CAD build for the part. Positions are in the model's coordinates, mm. Face numbers are marked on the shaded views. A direction names the side the tool comes from. Round coordinates to 2 decimals unless told otherwise and drop trailing zeros. Order: outer loops, then holes, each group sorted by start corner. A loop starts at its lowest first (then second) coordinate and runs counter-clockwise, first axis right, second up. Notation, with made-up numbers: M 12,-22 L 26,-22 A21 ccw 26,9 Z; hole C -25,-25 d11. An arc over 180 degrees is marked long. Put each result on its own line as item: value.
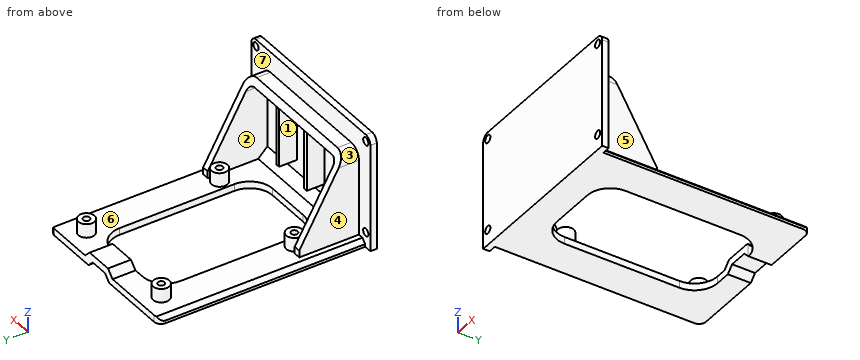
Autodesk Fusion 360 part; units mm, degrees
sketch "Sketch3" plane through (0, 0, 0) normal (0, 1, 0) x (1, 0, 0)
  line L0 (-39, -50) -> (39, -50)
  line L1 (39, -50) -> (39, 0)
  line L2 (39, 0) -> (-39, 0)
  line L3 (-39, 0) -> (-39, -50)
  line L4 (-56.129, 0) -> (56.129, 0) construction
  circle A0 centre (-36, -47) radius 1.7
  circle A1 centre (-36, -47) radius 3
  circle A2 centre (36, -47) radius 1.7
  circle A3 centre (36, -47) radius 3
  circle A4 centre (-36, -6.7) radius 1.7
  circle A5 centre (-36, -6.7) radius 3
  circle A6 centre (36, -6.7) radius 1.7
  circle A7 centre (36, -6.7) radius 3
  line L5 (-39, -5) -> (39, -5) construction
  dimension "d32" = 50
  dimension "d33" = 78
  dimension "d34" = 39
  dimension "d35" = 3.4
  dimension "d36" = 6
  dimension "d37" = 3.4
  dimension "d38" = 6
  dimension "d39" = 3.4
  dimension "d40" = 6
  dimension "d41" = 3.4
  dimension "d42" = 6
  dimension "d43" = 5
extrude "Extrude3" add sketch "Sketch3" along normal blind 3 contours A7 | A5 | L0 L1 L2 L3 A1 A3 | A1 | A3
sketch "Sketch4" plane through (0, 3, 0) normal (0, 1, 0) x (-1, 0, 0)
  circle A0 centre (36, 47) radius 1.7
  circle A1 centre (36, 6.7) radius 1.7
  circle A2 centre (-36, 47) radius 1.7
  circle A3 centre (-36, 6.7) radius 1.7
  line L0 (36, 50) -> (-36, 50)
  arc A4 (-36, 50) -> (-39, 47) centre (-36, 47) ccw
  line L1 (-39, 47) -> (-39, 0)
  line L2 (-39, 0) -> (39, 0)
  line L3 (39, 0) -> (39, 47)
  arc A5 (39, 47) -> (36, 50) centre (36, 47) ccw
  line L4 (-39, 3) -> (39, 3) construction
  line L5 (-35.6, 3) -> (35.6, 3)
  line L6 (35.6, 3) -> (35.6, 0)
  line L7 (35.6, 0) -> (-35.6, 0)
  line L8 (-35.6, 0) -> (-35.6, 3)
  line L9 (0, 50) -> (0, 0) construction
  line L10 (35.6, 1.2) -> (33.8, 3)
  line L11 (35.6, 1.2) -> (38.7868, 1.2) construction
  line L12 (-35.6, 1.2) -> (-33.8, 3)
  line L13 (-35.6, 1.2) -> (-32.9375, 1.2) construction
  point P0 (0, 3)
  dimension "d46" = 3
  dimension "d47" = 71.2
  dimension "d48" = 135
  dimension "d49" = 1.2
  dimension "d50" = 45
  dimension "d51" = 1.2
extrude "Extrude4" add sketch "Sketch4" along normal blind 90 contours L2 L5 L6 L7 L8 L10 L12
sketch "Sketch5" plane through (0, 0, 3) normal (0, 0, 1) x (-1, 0, 0)
  line L0 (33.8, -3) -> (-33.8, -3)
  line L1 (-33.8, -3) -> (-33.8, -93)
  line L2 (-33.8, -93) -> (33.8, -93)
  line L3 (33.8, -93) -> (33.8, -3)
  line L4 (0, -3) -> (0, -93) construction
  circle A0 centre (24.5, -26.5) radius 1.45
  circle A1 centre (24.5, -26.5) radius 3.5
  circle A2 centre (24.5, -84.5) radius 1.45
  circle A3 centre (24.5, -84.5) radius 3.5
  circle A4 centre (-24.5, -26.5) radius 1.45
  circle A5 centre (-24.5, -26.5) radius 3.5
  circle A6 centre (-24.5, -84.5) radius 1.45
  circle A7 centre (-24.5, -84.5) radius 3.5
  line L5 (28, -3) -> (-28, -3)
  line L6 (-28, -3) -> (-28, -88) construction
  line L7 (-28, -88) -> (28, -88) construction
  line L8 (28, -88) -> (28, -3) construction
  line L9 (20, -13) -> (-20, -13)
  line L10 (-20, -13) -> (-20, -83)
  line L11 (-20, -83) -> (20, -83)
  line L12 (20, -83) -> (20, -13)
  line L13 (33.8, -48) -> (-33.8, -48) construction
  line L14 (-28.5, -3) -> (-31.5, -3)
  line L15 (-31.5, -3) -> (-31.5, -29)
  line L16 (-31.5, -29) -> (-28.5, -29)
  line L17 (-28.5, -29) -> (-28.5, -3)
  point P0 (0, -88)
  point P1 (-28, -3)
  point P2 (0, -13)
  point P3 (20, -48)
  point P4 (-33.8, -48)
  point P5 (33.8, -48)
  dimension "d54" = 2.9
  dimension "d55" = 7
  dimension "d56" = 2.9
  dimension "d57" = 7
  dimension "d58" = 2.9
  dimension "d59" = 7
  dimension "d60" = 2.9
  dimension "d61" = 7
  dimension "d62" = 58
  dimension "d63" = 49
  dimension "d64" = 23.5
  dimension "d70" = 56
  dimension "d71" = 85
  dimension "d86" = 70
  dimension "d87" = 70
  dimension "d88" = 40
  dimension "d159" = 3
  dimension "d160" = 26
  dimension "d161" = 7
extrude "Extrude8" add sketch "Sketch5" along normal blind 38 contours L0 L14 L15 L16 L17
chamfer "Chamfer4" distance 20 distance2 35 1 edges at (30, 29, 41) measured on face at (30.5, 11.6667, 41)
mirror "Mirror1" about plane through (0, 0, 0) normal (1, 0, 0) of "Extrude8"
extrude "Extrude7" cut sketch "Sketch5" against normal blind 3 contours L9 L10 L11 L12
extrude "Extrude5" add sketch "Sketch5" along normal blind 6 contours A1 | A3 | A5 | A7
fillet "Fillet1" radius 3 2 edges at (35.6, 93, 0.6) (-35.6, 93, 0.6)
sketch "Sketch7" plane through (0, 0, 0) normal (0, -1, 0) x (1, 0, 0)
  circle A0 centre (-36, 47) radius 1.7
  circle A1 centre (-36, 6.7) radius 1.7
  circle A2 centre (36, 47) radius 1.7
  circle A3 centre (36, 6.7) radius 1.7
  line L0 (36, 50) -> (-36, 50)
  arc A4 (-36, 50) -> (-39, 47) centre (-36, 47) ccw
  line L1 (-39, 47) -> (-39, 0)
  line L2 (-39, 0) -> (39, 0)
  line L3 (39, 0) -> (39, 47)
  arc A5 (39, 47) -> (36, 50) centre (36, 47) ccw
  line L4 (-28, 50) -> (-28, 0) construction
  line L5 (28, 50) -> (28, 0) construction
  line L6 (19, 50) -> (19, 48.3878)
  line L7 (-39, 3) -> (39, 3) construction
  line L8 (-21, 9) -> (-28, 9)
  line L9 (28, 9) -> (21, 9)
  point P0 (-24.5, 9)
  point P1 (24.5, 9)
  dimension "d72" = 11
  dimension "d73" = 11
  dimension "d74" = 3
fillet "Fillet2" radius 10 4 edges at (-20, 13, 1.5) (20, 13, 1.5) (-20, 83, 1.5) (20, 83, 1.5)
sketch "Sketch8" plane through (0, 0, 0) normal (0, 0, -1) x (1, 0, 0)
  line L0 (-10, -13) -> (10, -13)
  arc A0 (20, -23) -> (10, -13) centre (10, -23) ccw
  line L1 (20, -23) -> (20, -73)
  arc A1 (10, -83) -> (20, -73) centre (10, -73) ccw
  line L2 (10, -83) -> (-10, -83)
  arc A2 (-20, -73) -> (-10, -83) centre (-10, -73) ccw
  line L3 (-20, -73) -> (-20, -23)
  arc A3 (-10, -13) -> (-20, -23) centre (-10, -23) ccw
  arc A4 (-35.6, -90) -> (-32.6, -93) centre (-32.6, -90) ccw
  line L4 (-32.6, -93) -> (32.6, -93)
  arc A5 (32.6, -93) -> (35.6, -90) centre (32.6, -90) ccw
  line L5 (35.6, -90) -> (35.6, -3)
  line L6 (35.6, -3) -> (39, -3)
  line L7 (39, -3) -> (39, 0)
  line L8 (39, 0) -> (-39, 0)
  line L9 (-39, 0) -> (-39, -3)
  line L10 (-39, -3) -> (-35.6, -3)
  line L11 (-35.6, -3) -> (-35.6, -90)
  line L12 (3.6, -93) -> (3.6, -80.0711) construction
  line L13 (7.6, -93) -> (-0.4, -93)
  line L14 (-0.4, -93) -> (-0.4, -73.9514)
  line L15 (-0.4, -73.9514) -> (7.6, -73.9514)
  line L16 (7.6, -73.9514) -> (7.6, -93)
  dimension "d166" = 8
  dimension "d167" = 32
extrude "Extrude9" cut sketch "Sketch8" against normal blind 2.8 contours L2 L4 L13 L14 L16
sketch "Sketch11" plane through (0, 0, 3) normal (0, 0, 1) x (-1, 0, 0)
  line L0 (28.5, -29) -> (28.5, -3)
  line L1 (28.5, -3) -> (-28.5, -3)
  line L2 (-28.5, -3) -> (-28.5, -29)
  line L3 (-28.5, -29) -> (-31.5, -29)
  line L4 (-31.5, -29) -> (-31.5, -3)
  line L5 (-31.5, -3) -> (-33.8, -3)
  line L6 (-33.8, -3) -> (-33.8, -92.7495)
  arc A0 (-33.8, -92.7495) -> (-32.6, -93) centre (-32.6, -90) ccw
  line L7 (-32.6, -93) -> (32.6, -93)
  arc A1 (32.6, -93) -> (33.8, -92.7495) centre (32.6, -90) ccw
  line L8 (33.8, -92.7495) -> (33.8, -3)
  line L9 (33.8, -3) -> (31.5, -3)
  line L10 (31.5, -3) -> (31.5, -29)
  line L11 (31.5, -29) -> (28.5, -29)
  circle A2 centre (-24.5, -26.5) radius 3.5
  circle A3 centre (24.5, -26.5) radius 3.5
  line L12 (-10, -13) -> (10, -13)
  arc A4 (20, -23) -> (10, -13) centre (10, -23) ccw
  line L13 (20, -23) -> (20, -73)
  arc A5 (10, -83) -> (20, -73) centre (10, -73) ccw
  line L14 (10, -83) -> (-10, -83)
  arc A6 (-20, -73) -> (-10, -83) centre (-10, -73) ccw
  line L15 (-20, -73) -> (-20, -23)
  arc A7 (-10, -13) -> (-20, -23) centre (-10, -23) ccw
  circle A8 centre (24.5, -84.5) radius 3.5
  circle A9 centre (-24.5, -84.5) radius 3.5
  line L16 (-7.6, -83) -> (-7.6, -93)
  line L17 (0.4, -93) -> (0.4, -83)
  line L18 (-9.6, -83) -> (-9.6, -93)
  line L19 (2.4, -93) -> (2.4, -83)
  dimension "d170" = 2
  dimension "d171" = 2
extrude "Extrude10" add sketch "Sketch11" along normal blind 3 contours L7 L14 L17 L19 | L7 L14 L16 L17 | L7 L14 L16 L18
chamfer "Chamfer5" distance 3 angle 45 2 edges at (-2.4, 88, 3) (9.6, 88, 3)
chamfer "Chamfer6" distance 4 angle 45 1 edges at (0, 3, 3)
chamfer "Chamfer7" distance 2.8 angle 45 2 edges at (7.6, 88, 0) (-0.4, 88, 0)
chamfer "Chamfer8" distance 35 distance2 20 1 edges at (-30, 29, 41) measured on face at (-30.5, 29, 15.6667)
sketch "Sketch13" plane through (28.5, 0, 0) normal (-1, 0, 0) x (0, -1, 0)
  line L0 (-7, 3) -> (-3, 7)
  line L1 (-3, 7) -> (-3, 41)
  line L2 (-3, 41) -> (-9, 41)
  line L3 (-9, 41) -> (-29, 6)
  line L4 (-29, 6) -> (-29, 3)
  line L5 (-29, 3) -> (-7, 3)
  line L6 (-3, 41) -> (-10.7143, 41)
  line L7 (-10.7143, 41) -> (-10.7143, 38)
  line L8 (-10.7143, 38) -> (-3, 38)
  line L9 (-3, 38) -> (-3, 41)
  dimension "d311" = 3
extrude "Extrude12" add sketch "Sketch13" along normal up to surface (57 mm away) contours L1 L2 L3 L6 L8 L9
sketch "Sketch14" plane through (0, 3, 0) normal (0, 1, 0) x (-1, 0, 0)
  line L0 (28.5, 38) -> (-28.5, 38)
  line L1 (-28.5, 38) -> (-28.5, 7)
  line L2 (-28.5, 7) -> (28.5, 7)
  line L3 (28.5, 7) -> (28.5, 38)
  line L4 (-10.85, 38) -> (-9.15, 38)
  line L5 (-9.15, 38) -> (-9.15, 12.3)
  line L6 (-9.15, 12.3) -> (-10.85, 12.3)
  line L7 (-10.85, 12.3) -> (-10.85, 38)
  line L8 (7.15, 38) -> (9.05, 38)
  line L9 (9.05, 38) -> (9.05, 12.3)
  line L10 (9.05, 12.3) -> (7.15, 12.3)
  line L11 (7.15, 12.3) -> (7.15, 38)
extrude "Extrude13" add sketch "Sketch14" along normal blind 7.8 contours L0 L8 L9 L10 L11 | L0 L4 L5 L6 L7
fillet "Fillet4" radius 5 2 edges at (-31.5, 6, 41) (31.5, 6, 41)
fillet "Fillet5" radius 3 2 edges at (28.5, 6.8571, 38) (-28.5, 6.8571, 38)
extrude "Extrude14" cut 1 faces at (-11.4895, 0, 33.3208) along direction (0, 1, 0) blind 0.2
equation "d34 = d33 / 2"
equation "d37 = d35"
equation "d38 = d36"
equation "d39 = d35"
equation "d40 = d36"
equation "d41 = d35"
equation "d42 = d36"
equation "d56 = d54"
equation "d57 = d55"
equation "d58 = d54"
equation "d59 = d55"
equation "d60 = d54"
equation "d61 = d55"
Item 1: Band-saw the part on D-D on x = 15.5. Give the cut face in (y, z), and give its area (3 significant figures).
Answers below:
outline: M 0.2,0 L 14.65,0 L 14.65,3 L 7,3 L 3,7 L 3,38 L 10.71,38 L 9,41 L 3,41 L 3,50 L 0.2,50 Z; M 81.35,0 L 93,0 L 93,3 L 81.35,3 Z
area: 238 mm²
Item 2: Probe line 1 along X through (y, z) = (1.15, 6.7); line 2 along Z through (x, y) = (-36, 1.5); line 3 along X through (y, z) = (26.5, 4.65). List the from-to ranges inside material, lowest first. Write a range as [from, to].
Answers below:
line 1: [-39, -37.7], [-34.3, 34.3], [37.7, 39]
line 2: [0, 5], [8.4, 45.3], [48.7, 50]
line 3: [-31.5, -28.5], [-28, -25.95], [-23.05, -21], [21, 23.05], [25.95, 28], [28.5, 31.5]
Item 3: Pin check, flat tips, straight feed: P1, Ø2.5, axis at x = 24.5, y = 26.5, coming from the -Z side; P2, Ø3, axis at x = -24, y = 26, coming from the +Z side; P3, Ø0.9, axis at x = 30.5, z = 4, coming from the +Y side; P4, Ø0.9, axis at y = 38, z = 1.5, coming from the +X side. Stop position of each tip, or through.
Answers below:
P1: z = 0
P2: z = 9
P3: y = 29
P4: x = 35.6
Item 4: Mould opens along Z. For the marked faces 1, 2, 3 and 4 say: pulls with the +Z half, pulls with the -Z half, needs draft (parallel to the pull), parting line crosses it, or undercut.
Answers below:
face 1: undercut
face 2: undercut
face 3: pulls with the +Z half
face 4: needs draft
Item 5: Band-saw the part on C-C on z = 20. Give the cut face in (x, y).
Answers below:
outline: M -39,0.2 L 39,0.2 L 39,3 L 31.5,3 L 31.5,21 L 28.5,21 L 28.5,3 L 10.85,3 L 10.85,10.8 L 9.15,10.8 L 9.15,3 L -7.15,3 L -7.15,10.8 L -9.05,10.8 L -9.05,3 L -28.5,3 L -28.5,21 L -31.5,21 L -31.5,3 L -39,3 Z
Item 6: Band-saw the part on A-A on y = 66. Give the cut face in (x, z).
Answers below:
outline: M -35.6,0 L -20,0 L -20,3 L -33.8,3 L -35.6,1.2 Z; M 20,0 L 35.6,0 L 35.6,1.2 L 33.8,3 L 20,3 Z
Item 7: Tool access for the marked faces 5, 6 and 7: list every direction of +Z, -Z, +X, -X, +Y, -Y with a clear straight run to the whole face (end or side of a thin tool).
Answers below:
face 5: +Z, +X, +Y
face 6: none
face 7: +Z, +Y
